Build history of the part. All positions in model axes, mm. Face numbers are marked on the shaded views. Round coordinates to 2 decimals unless told otherwise and drop trailing zeros. Loops run counter-clockwise (first coordinate to the right, second up) from the corner with the lowest first, then second, coordinate; pieces in that order, holes last. Notation, with made-up numbers: (66, 7.5) - (71, 7.5) arc R24 ccw to (71, 25.5) - close; hole circle Ø5 at (12, 75). An arc over 180 degrees is marked (long way). Use a Markdown table: item, result.
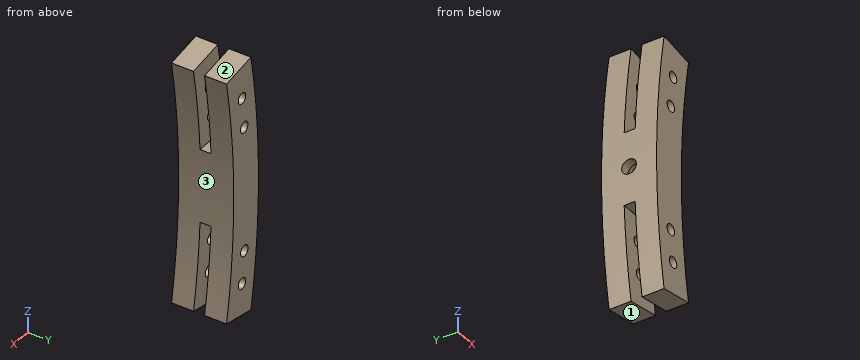
from build123d import *

# Parameters (mm, degrees)
BASE_DEPTH            = 7.5
MOUNT_START           = -1.5
MOUNT_DEPTH           = 3
MOUNT_HOLE_DEPTH      = 204.131478566
MOUNT_HOLE_DEPTH_BACK = 204.131478566
SKETCH12_R            = 1.5
SKETCH14_R            = 2
SHAFT_HOLE_DEPTH      = 37.394984425
SKETCH13_W            = 2.5
SKETCH13_H            = 3.5


with BuildPart() as part:
    # Sketch9 → base (new, symmetric)
    with BuildSketch(Plane(origin=(0, 0, 0), x_dir=(1, 0, 0), z_dir=(0, 1, 0))):
        with BuildLine():
            ThreePointArc((-187.113473072, -32.993153757), (-190, 0), (-187.113473072, 32.993153757))
            Line((-187.113473072, 32.993153757), (-196.961550602, 34.729635533))
            ThreePointArc((-196.961550602, 34.729635533), (-200, 0), (-196.961550602, -34.729635533))
            Line((-196.961550602, -34.729635533), (-187.113473072, -32.993153757))
        make_face()
    extrude(amount=BASE_DEPTH, both=True)

    # Sketch11 → mount (cut)
    with BuildSketch(Plane(origin=(0, 0, 0), x_dir=(1, 0, 0), z_dir=(0, 1, 0)).offset(MOUNT_START)):
        with BuildLine():
            Line((-189.73665961, -10), (-199.749843554, -10))
            ThreePointArc((-199.749843554, -10), (-198.7407137, -22.408228804), (-196.961550602, -34.729635533))
            Line((-196.961550602, -34.729635533), (-187.113473072, -32.993153757))
            ThreePointArc((-187.113473072, -32.993153757), (-188.775466906, -21.536552519), (-189.73665961, -10))
        make_face()
        with BuildLine():
            Line((-189.73665961, 10), (-199.749843554, 10))
            ThreePointArc((-199.749843554, 10), (-198.7407137, 22.408228804), (-196.961550602, 34.729635533))
            Line((-196.961550602, 34.729635533), (-187.113473072, 32.993153757))
            ThreePointArc((-187.113473072, 32.993153757), (-188.775466906, 21.536552519), (-189.73665961, 10))
        make_face()
    extrude(amount=MOUNT_DEPTH, mode=Mode.SUBTRACT)

    # Sketch12 → mount hole (cut, two sides: drawn at the far end of the back side and taken through both)
    with BuildSketch(Plane(origin=(0, 0, 0), x_dir=(1, 0, 0), z_dir=(0, 1, 0)).offset(-MOUNT_HOLE_DEPTH_BACK)):
        with Locations(Location((-193.331747968, 25.452607483, 0), (0, 0, 270))):
            Circle(SKETCH12_R)
        with Locations(Location((-194.257966128, 16.995369836, 0), (0, 0, 270))):
            Circle(SKETCH12_R)
        with Locations(Location((-194.257966128, -16.995369836, 0), (0, 0, 270))):
            Circle(SKETCH12_R)
        with Locations(Location((-193.331747968, -25.452607483, 0), (0, 0, 270))):
            Circle(SKETCH12_R)
    extrude(amount=MOUNT_HOLE_DEPTH + MOUNT_HOLE_DEPTH_BACK, mode=Mode.SUBTRACT)

    # Sketch14 → shaft hole (cut, through all)
    with BuildSketch(Plane.ZY.offset(195)):
        with Locations(Location((0, 0, 0), (0, 0, 90))):
            Circle(SKETCH14_R)
    extrude(amount=SHAFT_HOLE_DEPTH, mode=Mode.SUBTRACT)

    # Sketch13 → bearinghole (revolve, cut)
    with BuildSketch(Plane(origin=(0, 0, 0), x_dir=(1, 0, 0), z_dir=(0, 1, 0)), mode=Mode.PRIVATE) as bearinghole_sk:
        with Locations((-196.25, 1.75)):
            Rectangle(SKETCH13_W, SKETCH13_H)
    revolve(bearinghole_sk.sketch.rotate(Axis((0, 0, 0), (-1, 0, 0)), 270), axis=Axis((0, 0, 0), (-1, 0, 0)), mode=Mode.SUBTRACT)


solid = part.part
Q1. Cut at B-B, the plane z = 17. List the corners of the cut face in (x, y), plus the area to 3 significant figures.
Results found:
| item | result |
|---|---|
| outline | (-199.28, -7.5) - (-195.76, -7.5) - (-195.76, -1.5) - (-199.28, -1.5) - close; (-199.28, 1.5) - (-195.76, 1.5) - (-195.76, 7.5) - (-199.28, 7.5) - close; (-192.76, -7.5) - (-189.24, -7.5) - (-189.24, -1.5) - (-192.76, -1.5) - close; (-192.76, 1.5) - (-189.24, 1.5) - (-189.24, 7.5) - (-192.76, 7.5) - close |
| area | 84.5 mm2 |
Q2. Cut at A-A, the plane y = 0. List the corners of the cut face in (x, z).
Results found:
| item | result |
|---|---|
| outline | (-199.99, -2) arc R200 ccw to (-199.75, -10) - (-189.74, -10) arc R190 cw to (-189.74, 10) - (-199.75, 10) arc R200 ccw to (-199.99, 2) - (-197.5, 2) - (-197.5, 3.5) - (-195, 3.5) - (-195, -3.5) - (-197.5, -3.5) - (-197.5, -2) - close |
Q3. Pull direction Z, two halves, no side cores. Call the marked faces 1, 2 and 3: pulls with the +Z half, pulls with the -Z half, needs draft (parallel to the pull), parting line crosses it, or undercut.
Results found:
| item | result |
|---|---|
| face 1 | pulls with the -Z half |
| face 2 | pulls with the +Z half |
| face 3 | undercut |
Q4. Cut at C-C, the plane x = -188.5. List the corners of the cut face in (y, z).
Results found:
| item | result |
|---|---|
| outline | (-7.5, -33.24) - (-1.5, -33.24) - (-1.5, -23.83) - (-7.5, -23.83) - close; (-7.5, 23.83) - (-1.5, 23.83) - (-1.5, 33.24) - (-7.5, 33.24) - close; (1.5, -33.24) - (7.5, -33.24) - (7.5, -23.83) - (1.5, -23.83) - close; (1.5, 23.83) - (7.5, 23.83) - (7.5, 33.24) - (1.5, 33.24) - close |
Q5. Probe line 1 (Y direction, x = -197.25, z = 12); line 2 (Z direction, x = -193, y = 5.75); line 3 (Z direction, x = -198.35, y = 0). List the from-to ranges inside material, lowest first.
Results found:
| item | result |
|---|---|
| line 1 | y = -7.5 to -1.5, 1.5 to 7.5 |
| line 2 | z = -34.03 to -26.92, -23.99 to -17.81, -16.18 to 16.18, 17.81 to 23.99, 26.92 to 34.03 |
| line 3 | z = -10 to -2, 2 to 10 |
Q6. Drop flat-ended pins along their axis: pin 1 (2.5 mm diameter, centred on x = -192.5, y = -0.5, fed in from +Z); pin 2 (5 mm diameter, centred on y = -2, z = -1.5, fed in from +X); pin 3 (1.5 mm diameter, centred on x = -196, y = -0.5, fed in from -Z). Give the stop position or say it passes through.
Results found:
| item | result |
|---|---|
| pin 1 | stops at z = 34.08 |
| pin 2 | stops at x = -189.96 |
| pin 3 | stops at z = -10 |
Q7. Cut at D-D, the plane z = 0. List the corners of the cut face in (x, y), plus the area to 4 significant figures.
Results found:
| item | result |
|---|---|
| outline | (-200, -7.5) - (-190, -7.5) - (-190, 7.5) - (-200, 7.5) - (-200, 2) - (-197.5, 2) - (-197.5, 3.5) - (-195, 3.5) - (-195, -3.5) - (-197.5, -3.5) - (-197.5, -2) - (-200, -2) - close |
| area | 122.5 mm2 |
